```python
from build123d import *

# Parameters (mm, degrees)
F0_R      = 12.7
F1_DEPTH  = 60.325
F2_R      = 7.874
F4_DEPTH  = 19.05
F6_DEPTH  = 19.05
F7_R      = 5.08
F8_R      = 6.35
F9_DEPTH  = 22.353
F10_W     = 50.8
F10_H     = 22.3266
F11_DEPTH = 44.704
F12_R     = 3.302


with BuildPart() as f1:
    # F0 (on Front) → F1 (new body)
    with BuildSketch(Plane.XZ):
        with BuildLine():
            Line((194.2084, 0), (22.352, 0))
            ThreePointArc((22.352, 0), (15.8052507731, -15.8052507731), (0, -22.352))
            Line((0, -22.352), (194.2084, -22.352))
            Line((194.2084, -22.352), (194.2084, 0))
        make_face()
        with BuildLine():
            ThreePointArc((0, -22.352), (15.8052507731, -15.8052507731), (22.352, 0))
            ThreePointArc((22.352, 0), (-15.8052507731, 15.8052507731), (0, -22.352))
        make_face()
        Circle(F0_R, mode=Mode.SUBTRACT)
    extrude(amount=-F1_DEPTH)

    # F2
    f2_edges = [f1.edges().sort_by_distance(p)[0] for p in [
        (194.2084, 30.1625, 0),
    ]]
    fillet(f2_edges, radius=F2_R)

    # F3 (on face) → F4 (join)
    with BuildSketch(Plane.XZ):
        with BuildLine():
            ThreePointArc((131.0386, 34.798), (127.4644153616, 16.0823576341), (117.2464, 0))
            Line((117.2464, 0), (150.0886, 0))
            Line((150.0886, 0), (150.0886, 34.798))
            Line((150.0886, 34.798), (131.0386, 34.798))
        make_face()
    extrude(amount=-F4_DEPTH)

    # F5 (on face) → F6 (cut)
    with BuildSketch(Plane.XZ):
        Polygon((117.2464, -22.352), (117.2464, 0), (85.852, 0), (91.8464, -22.352), align=None)
    extrude(amount=-F6_DEPTH, mode=Mode.SUBTRACT)

    # F7
    f7_edges = [f1.edges().sort_by_distance(p)[0] for p in [
        (150.0886, 9.525, 34.798),
    ]]
    fillet(f7_edges, radius=F7_R)

    # F8 (on face) → F9 (cut, through all)
    with BuildSketch(Plane.XY):
        with Locations((155.3464, 37.973)):
            Circle(F8_R)
    extrude(amount=-F9_DEPTH, mode=Mode.SUBTRACT)

    # F10 (on face) → F11 (cut)
    with BuildSketch(Plane(origin=(0, 0, -22.352), x_dir=(1, 0, 0), z_dir=(0, 0, -1))):
        with Locations((3.048, -30.1625)):
            Rectangle(F10_W, F10_H)
    extrude(amount=-F11_DEPTH, mode=Mode.SUBTRACT)

    # F12
    f12_edges = [f1.edges().sort_by_distance(p)[0] for p in [
        (22.352, 9.4996, 0),
        (22.352, 50.8254, 0),
        (150.0886, 9.525, 0),
    ]]
    fillet(f12_edges, radius=F12_R)


solid = f1.part
```
Source: CAD feature listing. Evaluate the final solid. Frame: model axes, mm. A direction names the side the tool comes from. Round coordinates to 2 decimals unless told otherwise and drop trailing zeros. Write each loop counter-clockwise with the first axis right and the second up, starting at its lowest first coordinate (ties: lowest second). Pieces come first, ordered by that corner, then holes. Notation, with made-up numbers: M 30.25,-12.75 L 62.25,-12.75 A31 cw 62.25,12.25 Z; hole C 81,77 d4. An arc over 180 degrees is marked long. Answer as a JSON object with one key per item and string values. Group by question number.
(1) Ray query, line 1 (Z direction, x = -1, y = 3.5); line 2 (Y direction, x = 109.5, z = -18.5) (3 decimals); line 3 (Z direction, x = 10, y = 14). Return the intervals inside material, ascending. Write a range as [from, to].
(2) Mould query, pull axis Y, two halves, no side actions, for faces 1 (the cylindrical face through (-2.75, 50.69, -12.4)), 2 (the flat face through (28.448, 30, -11)), 3 (the flat face through (147, 0, 0)). Classes: +Y half, -Y half, draft (parallel to the pull), parting line (faces both ways), or undercut.
(3) Section query A-A on y = 10. Output: boundary loops of the cut face in (x, z), then the cut area to 3 significant figures.
(4) Section query B-B on z = -3. Output: boundary loops of the cut face in (x, y) (3 decimals), then the cut area to 3 significant figures.
(5) Section query C-C on y = 28.5. Output: boundary loops of the cut face in (x, z).
(6) First-contact query: pin 1 (5 mm diameter, centred on x = 57.5, y = 20, fed in from +Z); pin 2 (10 mm diameter, centred on x = 154, y = 12, fed in from +Z); pin 3 (5.5 mm diameter, centred on y = 5.5, z = 20, fed in from +X); pin 4 (15 mm diameter, centred on x = 0, z = 0, fed in from +Y). Flat tips, straight axial feed; report the tip coordinate or a pass-through.
(7) Section query D-D on z = 10.5. Output: boundary loops of the cut face in (x, y) (3 decimals).
(8) Reachability of faces 4 (the flat face through (88.8, 9.4, -11)), 5 (the flat face through (139, 19.05, 18)), 6 (the flat face through (8.3, 41.326, -10.2)) from +Z, -Z, +X, -X, +Y, -Y: full face, straight path, thin tool, end or side. Return the list, or none.
Computed values:
{
 "1": {"line 1": "[-22.33, -12.66], [12.66, 22.33]", "line 2": "[19.05, 60.325]", "line 3": "[-22.35, -7.83], [7.83, 19.99]"},
 "2": {"face 1": "draft", "face 2": "undercut", "face 3": "-Y half"},
 "3": {"outline": "M 0,-22.35 L 91.85,-22.35 L 85.85,0 L 25.44,0 A3.3 cw 22.17,2.88 A22.35 ccw long Z; M 117.25,-22.35 L 194.21,-22.35 L 194.21,-7.87 A7.87 ccw 186.33,0 L 153.39,0 A3.3 cw 150.09,3.3 L 150.09,29.72 A5.08 ccw 145.01,34.8 L 131.04,34.8 A50.8 cw 117.25,0 Z; hole C 0,0 d25.4", "area": "5,180 mm^2"},
 "4": {"outline": "M -22.15,0 L -12.341,0 L -12.341,18.999 L -22.15,18.999 Z; M -22.15,41.326 L -12.341,41.326 L -12.341,60.325 L -22.15,60.325 Z; M 12.341,0 L 86.657,0 L 86.657,19.05 L 117.246,19.05 L 117.246,0 L 192.519,0 L 192.519,60.325 L 12.341,60.325 L 12.341,41.326 L 28.448,41.326 L 28.448,18.999 L 12.341,18.999 Z; hole C 155.346,37.973 d12.7", "area": "10,200 mm^2"},
 "5": {"outline": "M 28.45,-22.35 L 194.21,-22.35 L 194.21,-7.87 A7.87 ccw 186.33,0 L 28.45,0 Z"},
 "6": {"pin 1": "z = 0", "pin 2": "z = 32.86", "pin 3": "x = 150.09", "pin 4": "through"},
 "7": {"outline": "M -19.732,0 L -7.144,0 L -7.144,18.999 L -19.732,18.999 Z; M -19.732,41.326 L -7.144,41.326 L -7.144,60.325 L -19.732,60.325 Z; M 7.144,0 L 19.732,0 L 19.732,18.999 L 7.144,18.999 Z; M 7.144,41.326 L 19.732,41.326 L 19.732,60.325 L 7.144,60.325 Z; M 124.85,0 L 150.089,0 L 150.089,19.05 L 124.85,19.05 Z"},
 "8": {"face 4": "+Z, -Y", "face 5": "+Z, +X, -X, +Y", "face 6": "+Z, -Z, -X"}
}
